Autodesk Inventor part; units mm, degrees
ref_plane "Work Plane2" through (68, 0, 0) normal (1, 0, 0) x (0, 1, 0)
ref_plane "XZ Plane" through (0, 0, 0) normal (0, 1, 0) x (-1, 0, 0)
ref_plane "XY Plane" through (0, 0, 0) normal (0, 0, 1) x (1, 0, 0)
sketch "Sketch1" plane through (0, 0, 0) normal (0, 0, 1) x (1, 0, 0)
  circle A0 centre (0, 0) radius 8
  dimension "d0" = 16
extrude "Extrusion1" add sketch "Sketch1" along normal blind 10
ref_plane "Work Plane1" through (8, 0, 0) normal (1, 0, 0) x (0, 1, 0)
sketch "Sketch2" plane through (8, 0, 0) normal (1, 0, 0) x (0, 1, 0)
  line L0 (8, 10) -> (-8, 10)
  line L1 (8, 0) -> (-8, 0)
  line L2 (8, 0) -> (-8, 0)
  line L3 (-8, 10) -> (8, 10)
  line L4 (8, 10) -> (8, 0)
  line L5 (8, 0) -> (-8, 0)
  line L6 (-8, 0) -> (-8, 10)
  line L7 (-8, 10) -> (8, 0) construction
  line L8 (8, 10) -> (-8, 0) construction
  point P0 (0, 0)
  point P1 (0, 5)
extrude "Extrusion2" add sketch "Sketch2" along normal blind 67 and the other way blind 8
sketch "Sketch3" plane through (0, 0, 0) normal (0, 0, -1) x (-1, 0, 0)
  line L0 (0, 0) -> (-75, 0)
  line L1 (-75, -8) -> (-75, 8)
  circle A0 centre (-75, 0) radius 8
  dimension "d8" = 75
extrude "Extrusion3" add sketch "Sketch3" against normal blind 10 contours L1 A0
sketch "Sketch4" plane through (0, 0, 0) normal (0, 0, -1) x (-1, 0, 0)
  line L0 (0, 0) -> (-75, 0)
  line L1 (0, -8) -> (-75, -8)
  line L2 (0, 0) -> (75, 0) construction
  circle A0 centre (-75, 0) radius 4
  circle A1 centre (0, 0) radius 4
  dimension "d11" = 75
  dimension "d12" = 180
  dimension "d14" = 8
  dimension "d15" = 8
extrude "Extrusion4" add sketch "Sketch4" along normal blind 20 contours A1
hole "Hole1" at (75, 0, 0) direction (0, 0, 1) diameter 8 end through all
ref_plane "Work Plane2" through (68, 0, 0) normal (1, 0, 0) x (0, 1, 0)
sketch "Sketch6" plane through (68, 0, 0) normal (1, 0, 0) x (0, 1, 0)
  line L0 (-8, 0) -> (-8, 10)
  line L1 (8, 7.5) -> (-8, 7.5)
  line L2 (-8, 7.5) -> (-8, 2.5)
  line L3 (-8, 2.5) -> (8, 2.5)
  line L4 (8, 2.5) -> (8, 7.5)
  line L5 (8, 7.5) -> (-8, 2.5) construction
  line L6 (-8, 7.5) -> (8, 2.5) construction
  point P0 (0, 0)
  point P1 (0, 5)
  dimension "d28" = 5
extrude "Extrusion6" [suppressed]
fillet "Fillet1" radius 2 8 edges at (-8, 0, 10) (37.5, -8, 10) (83, 0, 10) (37.5, 8, 10) (83, 0, 0) (37.5, -8, 0) (-8, 0, 0) (37.5, 8, 0)
properties part number "Manivela" material "Iron, Ductile"
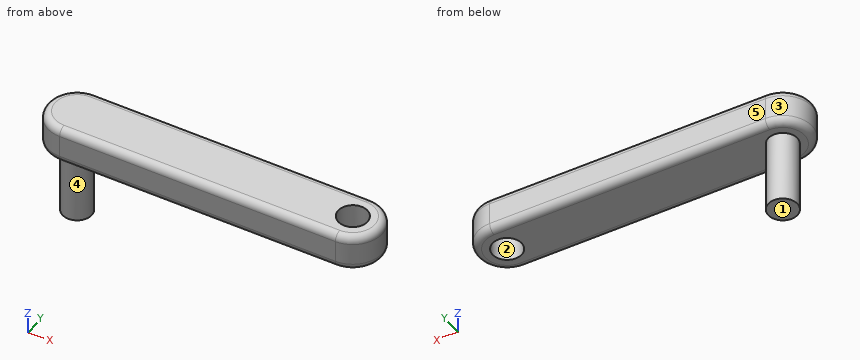
Part model, mm, in its own coordinate system. Face numbers are marked on the shaded views. A direction names the side the tool comes from. Give positions to 0.01 mm unless a question says otherwise; leave off trailing zeros. Order: outer loops, then holes, each group sorted by start corner. A loop starts at its lowest first (then second) coordinate and runs counter-clockwise, first axis right, second up. Notation, with made-up numbers: (73.5, 55) - (106.5, 55) arc R18 cw to (106.5, 80) - close; hole circle Ø8 at (7.5, 62.25). An arc over 180 degrees is marked (long way). Use a Markdown table: item, result.
1) Saw through at A-A on y = 0. List the corners of the cut face in (x, z), plus the area to 3 significant figures.
Checked values:
| item | result |
|---|---|
| outline | (-8, 2) arc R2 ccw to (-6, 0) - (-4, 0) - (-4, -20) - (4, -20) - (4, 0) - (71, 0) - (71, 10) - (-6, 10) arc R2 ccw to (-8, 8) - close; (79, 0) - (81, 0) arc R2 ccw to (83, 2) - (83, 8) arc R2 ccw to (81, 10) - (79, 10) - close |
| area | 987 mm² |
2) Probe L1, parallel to X at y = 0, z = 7.25; L2, parallel to Y at x = 75, z = 7.75; L3, parallel to Z at x = 32, y = -5.5. List the from-to ranges inside material, lowest first. Write a range as from..to.
Checked values:
| item | result |
|---|---|
| L1 | -8..71, 79..83 |
| L2 | -8..-4, 4..8 |
| L3 | 0..10 |
3) Two-plate mould, pull along X, no slides. Class the marked faces 1, 2 and 3: +X half, -X half, draft (parallel to the pull), parting line (faces both ways), or undercut.
Checked values:
| item | result |
|---|---|
| face 1 | draft |
| face 2 | undercut |
| face 3 | -X half |
4) Saw through at D-D on z = -5. List the corners of the cut face in (x, y), plus the area to 3 significant figures.
Checked values:
| item | result |
|---|---|
| outline | circle Ø8 at (0, 0) |
| area | 50.3 mm² |
5) Saw through at C-C on x = 68.5. List the corners of the cut face in (y, z), plus the area to 3 significant figures.
Checked values:
| item | result |
|---|---|
| outline | (-8, 2) arc R2 ccw to (-6, 0) - (6, 0) arc R2 ccw to (8, 2) - (8, 8) arc R2 ccw to (6, 10) - (-6, 10) arc R2 ccw to (-8, 8) - close |
| area | 157 mm² |
6) 3-axis set-ups, long thin cutter, end or side, ignore diameter. For the marked faces 4 and 5: which of +Z, -Z, +X, -X, +Y, -Y reach the whole face in a straight line?
Checked values:
| item | result |
|---|---|
| face 4 | -Z |
| face 5 | +Z, -Z, +X, -X, +Y |
7) Saw through at B-B on z = 3. List the corners of the cut face in (x, y), plus the area to 3 significant figures.
Checked values:
| item | result |
|---|---|
| outline | (0, -8) - (75, -8) arc R8 ccw to (75, 8) - (0, 8) arc R8 ccw to start; hole circle Ø8 at (75, 0) |
| area | 1,350 mm² |
8) Flat gauge pins, fed straight in: P1, Ø8, axis at y = 3.5, z = -13.5, coming from the -X side; P2, Ø6, axis at x = 8, y = 4, coming from the -Z side. Where does each tip first touch, or does it go through?
Checked values:
| item | result |
|---|---|
| P1 | x = -4 |
| P2 | z = 0 |
